Model file for the job. Use its own axes, mm. Face numbers are marked on the shaded views. A direction names the side the tool comes from. Round coordinates to 2 decimals unless told otherwise and drop trailing zeros. Loops run counter-clockwise (first coordinate to the right, second up) from the corner with the lowest first, then second, coordinate; pieces in that order, holes last.
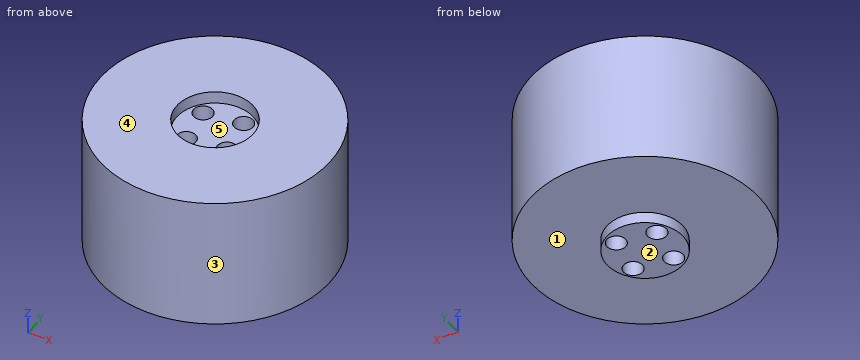
from build123d import *

# Parameters (mm, degrees)
SKETCH1_R           = 60
BOSS_EXTRUDE1_DEPTH = 70
SKETCH2_R           = 20.02
CUT_EXTRUDE1_DEPTH  = 6.5
SKETCH3_R           = 20
BOSS_EXTRUDE2_DEPTH = 6
SKETCH4_R           = 5
CUT_EXTRUDE2_DEPTH  = 114.912246927
CIRPATTERN1_COUNT   = 4


with BuildPart() as part:
    # Sketch1 → Boss-Extrude1 (new body)
    with BuildSketch(Plane.XY):
        Circle(SKETCH1_R)
    extrude(amount=BOSS_EXTRUDE1_DEPTH)

    # Sketch2 → Cut-Extrude1 (cut)
    with BuildSketch(Plane.XY.offset(70)):
        Circle(SKETCH2_R)
    extrude(amount=-CUT_EXTRUDE1_DEPTH, mode=Mode.SUBTRACT)

    # Sketch3 → Boss-Extrude2 (add)
    with BuildSketch(Plane(origin=(0, 0, 0), x_dir=(-1, 0, 0), z_dir=(0, 0, -1))):
        Circle(SKETCH3_R)
    extrude(amount=BOSS_EXTRUDE2_DEPTH)

    # Sketch4 → Cut-Extrude2 (cut, through all)
    with BuildSketch(Plane.XY.offset(70)):
        with Locations((-11.27834561, 8.294511456)):
            Circle(SKETCH4_R)
    cut_extrude2 = extrude(amount=-CUT_EXTRUDE2_DEPTH, mode=Mode.SUBTRACT)

    # CirPattern1: Cut-Extrude2 ×4 about axis
    cirpattern1_axis = Axis((0, 0, 0), (0, 0, 1))
    for i in range(1, CIRPATTERN1_COUNT):
        add(cut_extrude2.rotate(cirpattern1_axis, i * 360 / CIRPATTERN1_COUNT), mode=Mode.SUBTRACT)


solid = part.part
Q1. Flat gauge pins, fed straight in: P1, Ø10, axis at y = 26, z = 6.5, coming from the +X side (3 decimals); P2, Ø11.5, axis at x = -11.28, y = 8.29, coming from the +Z side; P3, Ø6, axis at y = 14.5, z = 58, coming from the -X side. Where does each tip first touch, or does it go through?
Q2. Slice it at C-C on z = 50. Give the cut face in (x, y).
Q3. Tool access for the marked faces 1 and 2: list every direction of +Z, -Z, +X, -X, +Y, -Y with a clear straight run to the whole face (end or side of a thin tool).
Q4. Slice it at B-B on y = 10. Give the cut face in (x, z).
Q5. Probe line 1 (Y direction, x = 0, z = 68.5); line 2 (Y direction, x = 7.5, z = 45); line 3 (Z direction, x = -31.5, y = 23). List the from-to ranges inside material, lowest first.
Q6. Slice it at A-A on x = 0. Give the cut face in (y, z).
Q7. Pull direction Y, two halves, no side cores. Call the marked faces 3, 4 and 5: pulls with the +Y half, pulls with the -Y half, needs draft (parallel to the pull), parting line crosses it, or undercut.
Q8. Slice it at D-D on y = 41. Give the cut face in (x, z), plus the area to 3 significant figures.
Reply:
1. P1: stops at x = 56.205
1. P2: stops at z = 63.5
1. P3: stops at x = -58.89
2. outline: circle Ø120 at (0, 0); hole circle Ø10 at (-11.28, 8.29); hole circle Ø10 at (-8.29, -11.28); hole circle Ø10 at (8.29, 11.28); hole circle Ø10 at (11.28, -8.29)
3. face 1: -Z
3. face 2: -Z, +X, -X, +Y, -Y
4. outline: (-59.16, 0) - (-17.32, 0) - (-17.32, -6) - (-15.98, -6) - (-15.98, 63.5) - (-17.34, 63.5) - (-17.34, 70) - (-59.16, 70) - close; (-6.58, -6) - (3.46, -6) - (3.46, 63.5) - (-6.58, 63.5) - close; (13.13, -6) - (17.32, -6) - (17.32, 0) - (59.16, 0) - (59.16, 70) - (17.34, 70) - (17.34, 63.5) - (13.13, 63.5) - close
5. line 1: y = -60 to -20.02, 20.02 to 60
5. line 2: y = -59.53 to -11.57, -5.02 to 6.34, 16.21 to 59.53
5. line 3: z = 0 to 70
6. outline: (-60, 0) - (-20, 0) - (-20, -6) - (20, -6) - (20, 0) - (60, 0) - (60, 70) - (20.02, 70) - (20.02, 63.5) - (-20.02, 63.5) - (-20.02, 70) - (-60, 70) - close
7. face 3: parting line crosses it
7. face 4: needs draft
7. face 5: undercut
8. outline: (-43.81, 0) - (43.81, 0) - (43.81, 70) - (-43.81, 70) - close
8. area: 6,130 mm2
